Geometry: see drawing. Coordinates: mm, zero at the bounding-box minimum. A direction names the side the tool comes from. Give positions to 0.01 mm unless a question says otherwise; leave off trailing zeros. Order: outer loops, then holes, each group sorted by start corner. A loop starts at its lowest first (then second) coordinate and runs counter-clockwise, first axis right, second up. Notation, with made-up numbers: M 76.25,-6 L 125.25,-6 A6 cw 125.25,4 Z; hole C 74.25,88.25 d9. An arc over 180 degrees is marked long. Answer as a JSON object with one key per item and string values. Group by question number.
1. Pin query (flat end, axial travel): P1, Ø8, axis at x = 27, y = 24.5, coming from the +Z side; P2, Ø12.5, axis at y = 12.5, z = 11.5, coming from the -X side; P3, Ø2.5, axis at x = 25, y = 15.5, coming from the -Z side; P4, Ø12, axis at x = 19, z = 44.5, coming from the -Y side. Return the tip coordinate at first contact, or that it passes through.
2. Section query A-A (z = 5). Output: boundary loops of the cut face in (x, y), plus the area to 3 significant figures.
3. Set-up query: the marked faces 1, 2, 3 and 4. Return all of +Z, -Z, +X, -X, +Y, -Y with unobstructed straight access to the full face (end or side cutting, diameter ignored); none if empty.
4. Section query B-B (x = 5). Output: boundary loops of the cut face in (y, z), plus the area to 3 significant figures.
5. Section query C-C (y = 15). Output: boundary loops of the cut face in (x, z), plus the area to 3 significant figures.
6. Material intervals for L1, parallel to Z at x = 5, y = 31; L2, parallel to Y at x = 25, z = 19.5, sorted ascending. Write a range as [from, to].
7. Section query D-D (z = 35). Output: boundary loops of the cut face in (x, y), plus the area to 4 significant figures.
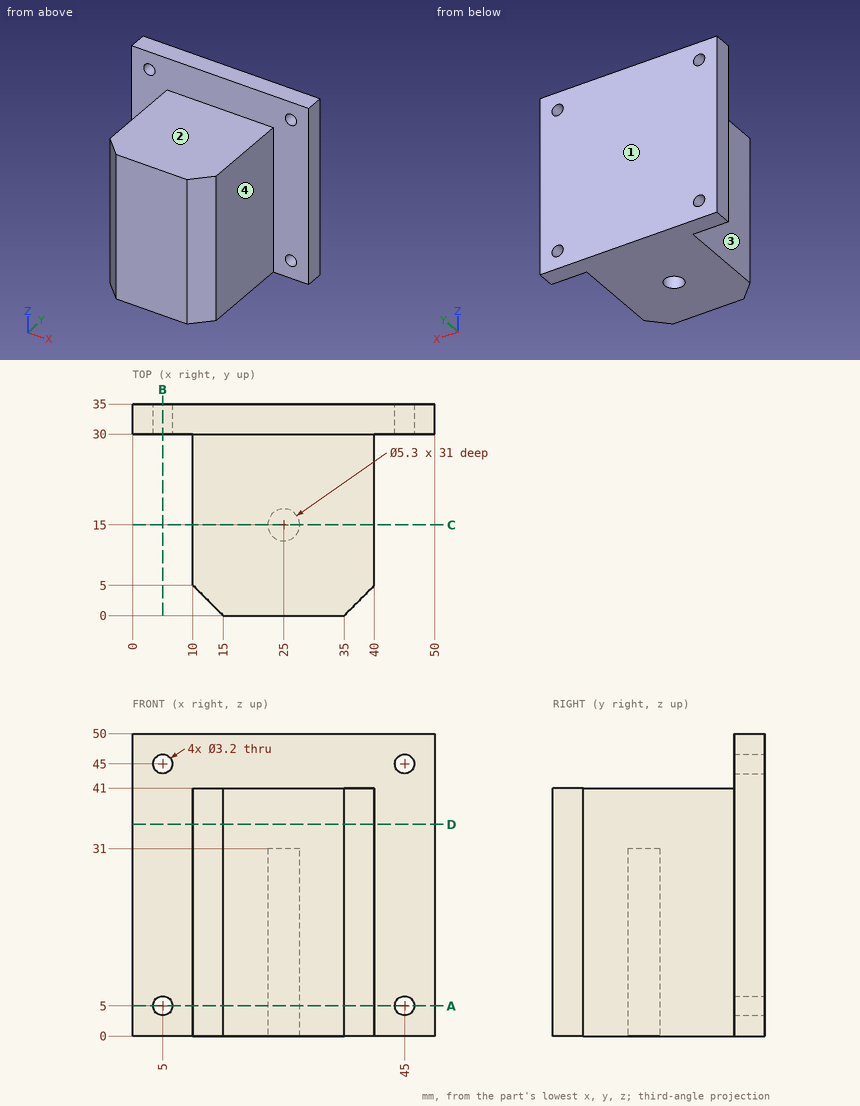
Answer sheet:
{
 "1": {"P1": "z = 41", "P2": "x = 10", "P3": "z = 31", "P4": "y = 0"},
 "2": {"outline": "M 0,30 L 3.4,30 L 3.4,35 L 0,35 Z; M 6.6,30 L 10,30 L 10,5 L 15,0 L 35,0 L 40,5 L 40,30 L 43.4,30 L 43.4,35 L 6.6,35 Z; M 46.6,30 L 50,30 L 50,35 L 46.6,35 Z; hole C 25,15 d5.3", "area": "1,070 mm^2"},
 "3": {"face 1": "+Z, -Z, +X, -X, +Y", "face 2": "+Z, +X, -X, -Y", "face 3": "+Z, -Z, -X, -Y", "face 4": "+Z, -Z, +X, -Y"},
 "4": {"outline": "M 30,0 L 35,0 L 35,3.4 L 30,3.4 Z; M 30,6.6 L 35,6.6 L 35,43.4 L 30,43.4 Z; M 30,46.6 L 35,46.6 L 35,50 L 30,50 Z", "area": "218 mm^2"},
 "5": {"outline": "M 10,0 L 22.35,0 L 22.35,31 L 27.65,31 L 27.65,0 L 40,0 L 40,41 L 10,41 Z", "area": "1,070 mm^2"},
 "6": {"L1": "[0, 3.4], [6.6, 43.4], [46.6, 50]", "L2": "[0, 12.35], [17.65, 35]"},
 "7": {"outline": "M 0,30 L 10,30 L 10,5 L 15,0 L 35,0 L 40,5 L 40,30 L 50,30 L 50,35 L 0,35 Z", "area": "1,125 mm^2"}
}
